Autodesk Inventor part; units mm, degrees
ref_plane "Work Plane1" through (0, -18.83, 0) normal (-1, 0, 0) x (0, 0, 1)
ref_plane "YZ Plane" through (0, 0, 0) normal (1, 0, 0) x (0, 1, 0)
ref_plane "XZ Plane" through (0, 0, 0) normal (0, 1, 0) x (-1, 0, 0)
sketch "Sketch1" plane through (0, 0, 0) normal (0, 0, 1) x (1, 0, 0)
  line L0 (-25, -25) -> (25, -25)
  line L1 (25, -25) -> (25, 25)
  line L2 (25, 25) -> (-25, 25)
  line L3 (-25, 25) -> (-25, -25)
  line L4 (-25, -25) -> (25, 25) construction
  line L5 (25, -25) -> (-25, 25) construction
  point P0 (0, 0)
  dimension "Width" = 50
  dimension "Height" = 50
extrude "Extrusion1" add sketch "Sketch1" along normal blind 6.35
sketch "Sketch2" plane through (0, 0, 6.35) normal (0, 0, 1) x (1, 0, 0)
  line L0 (-25, -25) -> (25, -25)
  line L1 (25, -25) -> (25, 25)
  line L2 (25, 25) -> (-25, 25)
  line L3 (-25, 25) -> (-25, -25)
  line L4 (0, 25) -> (0, -25) construction
  line L5 (-25, 0) -> (25, 0) construction
  point P0 (0, 0)
  point P1 (0, 0)
  point P2 (-10, 0)
  point P3 (0, 10)
  point P4 (0, -10)
  point P5 (10, 0)
  dimension "d4" = 10
  dimension "d5" = 10
  dimension "d6" = 10
  dimension "d7" = 10
hole "Hole1" at (0, 0, 6.35) at (-10, 0, 6.35) at (0, 10, 6.35) at (0, -10, 6.35) at (10, 0, 6.35) direction (0, 0, -1) diameter 5.02 end through all
sketch "Sketch3" plane through (0, 0, 6.35) normal (0, 0, 1) x (1, 0, 0)
  line L0 (-25, -25) -> (25, -25)
  line L1 (25, -25) -> (25, 25)
  line L2 (25, 25) -> (-25, 25)
  line L3 (-25, 25) -> (-25, -25)
  line L4 (0, 25) -> (0, -25) construction
  line L5 (25, 0) -> (-25, 0) construction
  line L6 (15, 25) -> (15, -25) construction
  line L7 (-25, -15) -> (25, -15) construction
  point P0 (15, 15)
  point P1 (-15, 15)
  dimension "d15" = 15
  dimension "d16" = 15
hole "Hole2" at (-15, 15, 6.35) at (15, 15, 6.35) direction (0, 0, -1) diameter 7.14 end through all counterbore diameter 12 counterbore depth 2.18
sketch "Sketch6" plane through (0, 0, 6.35) normal (0, 0, 1) x (1, 0, 0)
  circle A0 centre (-15, 15) radius 6
  circle A1 centre (15, 15) radius 6
  circle A2 centre (0, -10) radius 2.51
  circle A3 centre (-10, 0) radius 2.51
  circle A4 centre (0, 0) radius 2.51
  circle A5 centre (0, 10) radius 2.51
  circle A6 centre (10, 0) radius 2.51
  line L0 (-25, -25) -> (25, -25)
  line L1 (25, -25) -> (25, 25)
  line L2 (25, 25) -> (-25, 25)
  line L3 (-25, 25) -> (-25, -25)
sketch "Sketch7" plane through (0, 0, 6.35) normal (0, 0, 1) x (1, 0, 0)
  circle A0 centre (-15, 15) radius 6
  circle A1 centre (15, 15) radius 6
  line L0 (-25, -25) -> (25, -25)
  line L1 (25, -25) -> (25, 25)
  line L2 (-25, 25) -> (-25, -25)
  line L3 (15, 15) -> (15, -25) construction
  line L4 (25, -16.9) -> (-25, -16.9) construction
  line L5 (-15, 15) -> (-15, -16.9) construction
  point P0 (15, -16.9)
  dimension "d35" = 31.9
hole "Hole3" at (-15, -16.9, 6.35) at (15, -16.9, 6.35) direction (0, 0, -1) diameter 5 end through all counterbore diameter 10.1 counterbore depth 2
fillet "Fillet1" radius 6.17 4 edges at (25, 25, 3.175) (25, -25, 3.175) (-25, 25, 3.175) (-25, -25, 3.175)
sketch "Sketch4" plane through (0, 0, 6.35) normal (0, 0, 1) x (1, 0, 0)
  line L0 (25, -18.83) -> (25, 18.83)
  line L1 (-25, 18.83) -> (-25, -18.83)
  line L2 (-25, 0) -> (25, 0) construction
  line L3 (-22.25, 3.35) -> (-19.75, 3.35)
  line L4 (-19.75, 3.35) -> (-19.75, -3.35)
  line L5 (-19.75, -3.35) -> (-22.25, -3.35)
  line L6 (-22.25, -3.35) -> (-22.25, 3.35)
  line L7 (-22.25, 3.35) -> (-19.75, -3.35) construction
  line L8 (-19.75, 3.35) -> (-22.25, -3.35) construction
  point P0 (-21, 0)
  dimension "d25" = 2.5
  dimension "d27" = 5.25
  dimension "d28" = 6.7
extrude "Extrusion2" cut sketch "Sketch4" against normal through all
sketch "Sketch5" plane through (-25, -18.83, 0) normal (-1, 0, 0) x (0, 0, 1)
  line L0 (6.35, 37.66) -> (6.35, 0)
  line L1 (0, 15.48) -> (0, 22.18)
  line L2 (6.35, 22.18) -> (0, 22.18)
  line L3 (6.35, 15.48) -> (0, 15.48)
  line L4 (6.35, 22.18) -> (4.17, 22.18)
  line L5 (4.17, 22.18) -> (4.17, 15.48)
  line L6 (4.17, 15.48) -> (6.35, 15.48)
  line L7 (6.35, 15.48) -> (6.35, 22.18)
  point P0 (0, 18.83)
  dimension "d31" = 2.18
extrude "Extrusion3" cut sketch "Sketch5" against normal up to surface (5.25 mm away) contours L0 L3 L5 L2
ref_plane "Work Plane1" through (0, -18.83, 0) normal (-1, 0, 0) x (0, 0, 1)
mirror "Mirror1" about plane through (0, -18.83, 0) normal (-1, 0, 0) of "Extrusion2", "Extrusion3"
properties part number "Micro V Plate" material "Aluminum 6061"
Can you work these out from the model? Positions are in its coordinate system, mm. A direction names the side the tool comes from. Coordinates: 2 decimals unless noted, no trailing zeros. Loops run counter-clockwise (first coordinate to the right, second up) from the corner with the lowest first, then second, coordinate; pieces in that order, holes last.
Item 1: Suppose I cut it at D-D (x = 15). Please give me the cut outline in (y, z), then the cut area to 3 significant figures.
Answers below:
outline: (-25, 0) - (-19.4, 0) - (-19.4, 4.35) - (-21.95, 4.35) - (-21.95, 6.35) - (-25, 6.35) - close; (-14.4, 0) - (11.43, 0) - (11.43, 4.17) - (9, 4.17) - (9, 6.35) - (-11.85, 6.35) - (-11.85, 4.35) - (-14.4, 4.35) - close; (18.57, 0) - (25, 0) - (25, 6.35) - (21, 6.35) - (21, 4.17) - (18.57, 4.17) - close
area: 220 mm2
Item 2: Suppose I cut it at B-B (z = 2.5). State how many separate pieces and enclosed holes the cut face has, then the cut area to 3 significant figures.
Answers below:
separate pieces: 1
enclosed holes: 11
area: 2,220 mm2
Item 3: Suppose I cut it at A-A (y = 0). Please give me the cut outline in (x, z), then the cut area to 3 significant figures.
Answers below:
outline: (-25, 0) - (-22.25, 0) - (-22.25, 4.17) - (-25, 4.17) - close; (-19.75, 0) - (-12.51, 0) - (-12.51, 6.35) - (-19.75, 6.35) - close; (-7.49, 0) - (-2.51, 0) - (-2.51, 6.35) - (-7.49, 6.35) - close; (2.51, 0) - (7.49, 0) - (7.49, 6.35) - (2.51, 6.35) - close; (12.51, 0) - (19.75, 0) - (19.75, 6.35) - (12.51, 6.35) - close; (22.25, 0) - (25, 0) - (25, 4.17) - (22.25, 4.17) - close
area: 178 mm2
Item 4: Please list where these lines run through material, in increasing order: L1, parallel to Y at x = 0, z = 2.5; L2, parallel to Y at x = 15, z = 4.85; L3, parallel to X at y = 0, z = 4.5.
Answers below:
L1: y = -25 to -12.51, -7.49 to -2.51, 2.51 to 7.49, 12.51 to 25
L2: y = -25 to -21.95, -11.85 to 9, 21 to 25
L3: x = -19.75 to -12.51, -7.49 to -2.51, 2.51 to 7.49, 12.51 to 19.75
Item 5: Suppose I cut it at C-C (x = 0). Please give me the cut outline in (y, z), then the cut area to 3 significant figures.
Answers below:
outline: (-25, 0) - (-12.51, 0) - (-12.51, 6.35) - (-25, 6.35) - close; (-7.49, 0) - (-2.51, 0) - (-2.51, 6.35) - (-7.49, 6.35) - close; (2.51, 0) - (7.49, 0) - (7.49, 6.35) - (2.51, 6.35) - close; (12.51, 0) - (25, 0) - (25, 6.35) - (12.51, 6.35) - close
area: 222 mm2
Item 6: I'm going to push flat-ended pins straight in: pin 1 (9.5 mm diameter, centred on x = -15, y = 15, fed in from +Z); pin 2 (6.5 mm diameter, centred on x = 15, y = -16.9, fed in from +Z). Where does each tip first touch, or does it pass through?
Answers below:
pin 1: stops at z = 4.17
pin 2: stops at z = 4.35
Item 7: If we mould it in two halves opening along X, with no side actions, what happens to faces 5 (the face through (-25, 0, 3)), 6 (the face through (24, 0, 4.17)), 7 (the face through (-22.25, 0, 2))? For each: released by +X, released by -X, zero draft, split by the parting line, or undercut.
Answers below:
face 5: released by -X
face 6: zero draft
face 7: undercut
Item 8: Which directions (+Z, -Z, +X, -X, +Y, -Y) give clear straight access to the entire face, cutting with the end or side of a thin tool? Please do faces 1 (the face through (-24, 0, 4.17)), 2 (the face through (22, -3.35, 4)), 3 (the face through (19.75, 0, 3)), 4 (the face through (23.145, -23.241, 3.219)).
Answers below:
face 1: +Z, -X
face 2: +Z
face 3: +Z, -Z
face 4: +Z, -Z, +X, -Y
